Check sheet for the modelled part. Datum: model origin and axes. Units: mm. Face numbers are marked on the shaded views. Give positions to 0.01 mm unless a question says otherwise; leave off trailing zeros. Order: outer loops, then holes, each group sorted by start corner. A loop starts at its lowest first (then second) coordinate and runs counter-clockwise, first axis right, second up. Notation, with made-up numbers: M -5,8.25 L 3,8.25 A16 ccw 3,16.25 Z; hole C -27,6 d7. An arc over 180 degrees is marked long. One line per question, with ' | ' between items. Start each with the question number.
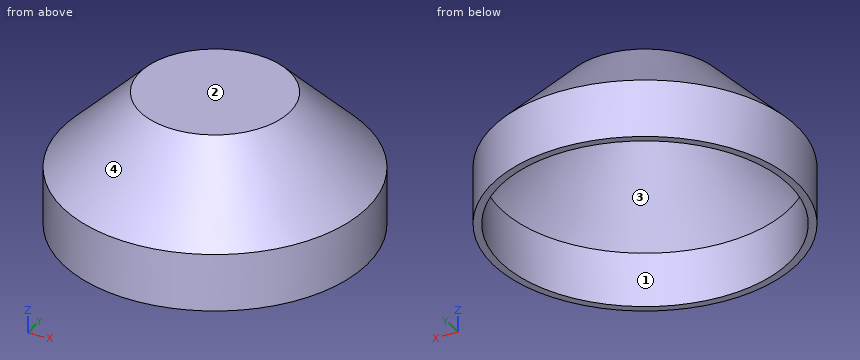
```python
from build123d import *

# Parameters (mm, degrees)
F0_R          = 39.385
F1_DEPTH      = 25
F1_DEPTH_BACK = 10
F2_SIZE       = 20
F3_T          = -2


with BuildPart() as f1:
    # F0 (on Top) → F1 (new body, two sides)
    with BuildSketch(Plane.XY) as f1_sk:
        Circle(F0_R)
    extrude(amount=F1_DEPTH)
    extrude(f1_sk.sketch, amount=-F1_DEPTH_BACK)

    # F2
    f2_edges = [f1.edges().sort_by_distance(p)[0] for p in [
        (-39.385, 0, 25),
    ]]
    chamfer(f2_edges, length=F2_SIZE)

    # F3
    f3_openings = [f1.faces().sort_by_distance(p)[0] for p in [
        (0, 0, -10),
    ]]
    offset(amount=F3_T, openings=f3_openings)


solid = f1.part
```
Item 1: Go/stop test with flat-tipped pins: P1, Ø4, axis at x = -25.5, z = 5, coming from the +Y side; P2, Ø1.5, axis at y = -8.5, z = 17.5, coming from the +X side; P3, Ø3, axis at y = 4.5, z = 19.5, coming from the -X side. Record where each tip stops, or that it passes through.
Item 2: Section check D-D, the plane z = 20. Record the cut outline in (x, y) (3 decimals).
Item 3: Scan lines: probe 1 along Y at (x, z) = (0, -5) (3 decimals); probe 2 along Z at (x, y) = (-15.5, -3); probe 3 along Y at (x, z) = (15, 22.5). Record each from-to range of solid material in increasing order. Write a range as [from, to].
Item 4: Draft check along Y on the marked faces 1, 2, 3 and 4. Enter one of: released by +Y, released by -Y, zero draft, split by the parting line, or undercut.
Item 5: Section check C-C, the plane z = 0.5. Record the cut outline in (x, y) (3 decimals), then the cut area to 3 significant figures.
Item 6: Section check A-A, the plane y = 0. Record the cut outline in (x, z) (3 decimals).
Reported:
1) P1: stops at y = 31.61 | P2: stops at x = 26.33 | P3: stops at x = -26.02
2) outline: C 0,0 d48.77; hole C 0,0 d43.113
3) probe 1: y = [-39.385, -37.385], [37.385, 39.385] | probe 2: z = [23, 25] | probe 3: y = [-15.94, -11.75], [11.75, 15.94]
4) face 1: undercut | face 2: zero draft | face 3: undercut | face 4: split by the parting line
5) outline: C 0,0 d78.77; hole C 0,0 d74.77 | area: 482 mm^2
6) outline: M -39.385,-10 L -37.385,-10 L -37.385,4.172 L -18.557,23 L 18.557,23 L 37.385,4.172 L 37.385,-10 L 39.385,-10 L 39.385,5 L 19.385,25 L -19.385,25 L -39.385,5 Z
